```python
from build123d import *

# Parameters (mm, degrees)
SKETCH1_W           = 282
SKETCH1_H           = 170
BOSS_EXTRUDE1_DEPTH = 60
CUT_EXTRUDE4_DEPTH  = 5
SKETCH8_W           = 160
SKETCH8_H           = 50
CUT_EXTRUDE5_DEPTH  = 279
CUT_EXTRUDE6_DEPTH  = 5
SKETCH10_R          = 5
CUT_EXTRUDE7_DEPTH  = 5
CUT_EXTRUDE8_DEPTH  = 5
CUT_EXTRUDE9_START  = -5
CUT_EXTRUDE9_DEPTH  = 5
SKETCH14_W          = 185
SKETCH14_H          = 5
BOSS_EXTRUDE2_DEPTH = 10
SKETCH15_W          = 185
SKETCH15_H          = 5
BOSS_EXTRUDE3_DEPTH = 10
SKETCH16_W          = 97
SKETCH16_H          = 15
CUT_EXTRUDE10_DEPTH = 170
BOSS_EXTRUDE4_DEPTH = 160
SKETCH18_W          = 15
SKETCH18_H          = 10
CUT_EXTRUDE11_DEPTH = 340.888216918
BOSS_EXTRUDE5_REACH = 339.267
SKETCH19_W          = 5
SKETCH19_H          = 50


with BuildPart() as part:
    # Sketch1 → Boss-Extrude1 (new body)
    with BuildSketch(Plane(origin=(0, 0, 0), x_dir=(1, 0, 0), z_dir=(0, 1, 0))):
        with Locations((141, 85)):
            Rectangle(SKETCH1_W, SKETCH1_H)
    extrude(amount=BOSS_EXTRUDE1_DEPTH)

    # Sketch7 → Cut-Extrude4 (cut)
    with BuildSketch(Plane.XZ):
        with BuildLine():
            Line((13.5, -37.5), (13.5, -132.5))
            ThreePointArc((13.5, -132.5), (11, -135), (8.5, -132.5))
            Line((8.5, -132.5), (8.5, -37.5))
            ThreePointArc((8.5, -37.5), (11, -35), (13.5, -37.5))
        make_face()
        with BuildLine():
            Line((58.5, -37.5), (58.5, -132.5))
            ThreePointArc((58.5, -132.5), (56, -135), (53.5, -132.5))
            Line((53.5, -132.5), (53.5, -37.5))
            ThreePointArc((53.5, -37.5), (56, -35), (58.5, -37.5))
        make_face()
        with BuildLine():
            Line((28.5, -37.5), (28.5, -132.5))
            ThreePointArc((28.5, -132.5), (26, -135), (23.5, -132.5))
            Line((23.5, -132.5), (23.5, -37.5))
            ThreePointArc((23.5, -37.5), (26, -35), (28.5, -37.5))
        make_face()
        with BuildLine():
            Line((43.5, -37.5), (43.5, -132.5))
            ThreePointArc((43.5, -132.5), (41, -135), (38.5, -132.5))
            Line((38.5, -132.5), (38.5, -37.5))
            ThreePointArc((38.5, -37.5), (41, -35), (43.5, -37.5))
        make_face()
    extrude(amount=-CUT_EXTRUDE4_DEPTH, mode=Mode.SUBTRACT)

    # Sketch8 → Cut-Extrude5 (cut)
    with BuildSketch(Plane(origin=(282, 0, 0), x_dir=(0, 0, -1), z_dir=(1, 0, 0))):
        with Locations((85, 30)):
            Rectangle(SKETCH8_W, SKETCH8_H)
    extrude(amount=-CUT_EXTRUDE5_DEPTH, mode=Mode.SUBTRACT)

    # Sketch9 → Cut-Extrude6 (cut)
    with BuildSketch(Plane.XY):
        Polygon((217.15, 25.8), (227.05, 25.8), (227.05, 8.15), (224.8, 5), (219.4, 5), (217.15, 8.15), align=None)
        Polygon((162.25, 25.8), (172.15, 25.8), (172.15, 8.15), (169.9, 5), (164.5, 5), (162.25, 8.15), align=None)
    extrude(amount=-CUT_EXTRUDE6_DEPTH, mode=Mode.SUBTRACT)

    # Sketch10 → Cut-Extrude7 (cut)
    with BuildSketch(Plane.ZY):
        with Locations((-129.202249563, 20)):
            Circle(SKETCH10_R)
        with Locations((-114.202249563, 20)):
            Circle(SKETCH10_R)
        with Locations((-99.202249563, 20)):
            Circle(SKETCH10_R)
        with Locations((-43.390057257, 20)):
            Circle(SKETCH10_R)
        with Locations((-58.390057257, 20)):
            Circle(SKETCH10_R)
        with Locations((-73.390057257, 20)):
            Circle(SKETCH10_R)
    extrude(amount=-CUT_EXTRUDE7_DEPTH, mode=Mode.SUBTRACT)

    # Sketch11 → Cut-Extrude8 (cut)
    with BuildSketch(Plane.XY):
        with BuildLine():
            Line((11, 13.5), (56, 13.5))
            ThreePointArc((56, 13.5), (58.5, 11), (56, 8.5))
            Line((56, 8.5), (11, 8.5))
            ThreePointArc((11, 8.5), (8.5, 11), (11, 13.5))
        make_face()
        with BuildLine():
            Line((11, 23.5), (56, 23.5))
            ThreePointArc((56, 23.5), (58.5, 21), (56, 18.5))
            Line((56, 18.5), (11, 18.5))
            ThreePointArc((11, 18.5), (8.5, 21), (11, 23.5))
        make_face()
    extrude(amount=-CUT_EXTRUDE8_DEPTH, mode=Mode.SUBTRACT)

    # Sketch12 → Cut-Extrude9 (cut)
    with BuildSketch(Plane(origin=(0, 0, -170), x_dir=(-1, 0, 0), z_dir=(0, 0, -1)).offset(CUT_EXTRUDE9_START)):
        with BuildLine():
            Line((-56, 13.5), (-11, 13.5))
            ThreePointArc((-11, 13.5), (-8.5, 11), (-11, 8.5))
            Line((-11, 8.5), (-56, 8.5))
            ThreePointArc((-56, 8.5), (-58.5, 11), (-56, 13.5))
        make_face()
        with BuildLine():
            Line((-56, 23.5), (-11, 23.5))
            ThreePointArc((-11, 23.5), (-8.5, 21), (-11, 18.5))
            Line((-11, 18.5), (-56, 18.5))
            ThreePointArc((-56, 18.5), (-58.5, 21), (-56, 23.5))
        make_face()
    extrude(amount=CUT_EXTRUDE9_DEPTH, mode=Mode.SUBTRACT)

    # Sketch14 → Boss-Extrude2 (add)
    with BuildSketch(Plane.XY):
        with Locations((189.5, 57.5)):
            Rectangle(SKETCH14_W, SKETCH14_H)
    extrude(amount=BOSS_EXTRUDE2_DEPTH)

    # Sketch15 → Boss-Extrude3 (add)
    with BuildSketch(Plane(origin=(0, 0, -170), x_dir=(-1, 0, 0), z_dir=(0, 0, -1))):
        with Locations((-189.5, 57.5)):
            Rectangle(SKETCH15_W, SKETCH15_H)
    extrude(amount=BOSS_EXTRUDE3_DEPTH)

    # Sketch16 → Cut-Extrude10 (cut)
    with BuildSketch(Plane.XY):
        with Locations((48.5, 52.5)):
            Rectangle(SKETCH16_W, SKETCH16_H)
    extrude(amount=-CUT_EXTRUDE10_DEPTH, mode=Mode.SUBTRACT)

    # Sketch17 → Boss-Extrude4 (add)
    with BuildSketch(Plane.XY.offset(-165)):
        Polygon((3, 45), (97, 45), (97, 55), (102, 55), (102, 40), (3, 40), align=None)
    extrude(amount=BOSS_EXTRUDE4_DEPTH)

    # Sketch18 → Cut-Extrude11 (cut, through all)
    with BuildSketch(Plane.XY):
        with Locations((69.5, 22)):
            Rectangle(SKETCH18_W, SKETCH18_H)
    extrude(amount=-CUT_EXTRUDE11_DEPTH, mode=Mode.SUBTRACT)

    # Sketch19 → Boss-Extrude5 (add, up to next)
    with BuildSketch(Plane.XY.offset(-165), mode=Mode.PRIVATE) as boss_extrude5_sk1:
        with Locations((279.5, 30)):
            Rectangle(SKETCH19_W, SKETCH19_H)
    boss_extrude5_tool1 = extrude(boss_extrude5_sk1.sketch, amount=BOSS_EXTRUDE5_REACH, mode=Mode.PRIVATE) - part.part
    add(boss_extrude5_tool1.solids().sort_by_distance((279.5, 30, -165))[0])


solid = part.part
```
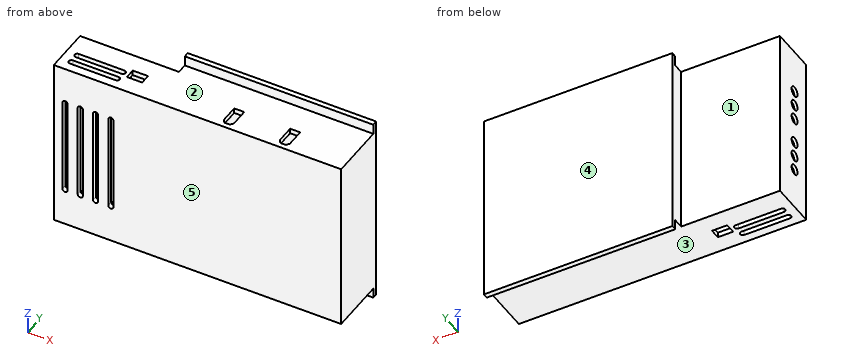
Build history of the part. All positions in model axes, mm. Face numbers are marked on the shaded views. A direction names the side the tool comes from. Give positions to 0.01 mm unless a question says otherwise; leave off trailing zeros. Loops run counter-clockwise (first coordinate to the right, second up) from the corner with the lowest first, then second, coordinate; pieces in that order, holes last.
Item 1: Which spindle directions (+Z, -Z, +X, -X, +Y, -Y) get a long thin tool onto all of the face, cutting with end or side? Do the marked faces 1, 2, 3, 4 and 5. Say none if no direction does.
Answers follow:
face 1: +Z, -Z, -X, +Y
face 2: +Z, +X, -X, -Y
face 3: -Z, +X, -X, -Y
face 4: +Z, -Z, +X, -X, +Y
face 5: +Z, -Z, +X, -X, -Y
Item 2: Drill centre lines: line 1 (Z direction, x = 120, y = 21.5); line 2 (Y direction, x = 18, z = -135.5); line 3 (Y direction, x = 185.5, z = -88). Where is each one in solid material? Low to high.
Answers follow:
line 1: z = -170 to -165, -5 to 0
line 2: y = 0 to 5, 40 to 45
line 3: y = 0 to 5, 55 to 60
Item 3: Slice it at C-C, the plane y = 36. List the corners of the cut face in (x, z).
Answers follow:
outline: (0, -170) - (282, -170) - (282, 0) - (0, 0) - close; hole (3, -165) - (277, -165) - (277, -5) - (3, -5) - close
Item 4: Flat gauge pins, fed straight in: pin 1 (12 mm diameter, centred on x = 240.5, y = 7.5, fed in from +Z); pin 2 (2 mm diameter, centred on x = 56.5, y = 30.5, fed in from -Z); pin 3 (2 mm diameter, centred on x = 45, y = 10.5, fed in from -Z); pin 4 (8 mm diameter, centred on y = 20, z = -99.2, fed in from -X). Where does each tip first touch, or does it go through?
Answers follow:
pin 1: stops at z = 0
pin 2: stops at z = -170
pin 3: passes through
pin 4: stops at x = 277
Item 5: Slice it at B-B, the plane x = 202. List the corners of the cut face in (y, z).
Answers follow:
outline: (0, -170) - (55, -170) - (55, -180) - (60, -180) - (60, 10) - (55, 10) - (55, 0) - (0, 0) - close; hole (5, -165) - (55, -165) - (55, -5) - (5, -5) - close
Item 6: Slice it at D-D, the plane z = -43. Give the number of separate pieces and of enclosed holes in the cut face, and give its area (3 significant figures).
Answers follow:
separate pieces: 5
enclosed holes: 0
area: 3,120 mm2
Item 7: Slice it at A-A, the plane y = 50.5. List the corners of the cut face in (x, z), and give its area (3 significant figures).
Answers follow:
outline: (97, -170) - (282, -170) - (282, 0) - (97, 0) - close; hole (102, -165) - (277, -165) - (277, -5) - (102, -5) - close
area: 3,450 mm2
